from build123d import *

# Parameters (mm, degrees)
SKETCH_1_R      = 7.75
SKETCH_1_R_2    = 1.15
EXTRUDE_1_DEPTH = 11
EXTRUDE_2_DEPTH = 35.9
SKETCH_3_R      = 2
EXTRUDE_3_DEPTH = 10


with BuildPart() as part:
    # 草图1 → 凸台-拉伸1 (new body)
    with BuildSketch(Plane.XY):
        Circle(SKETCH_1_R)
        with Locations((4.353856496, 0)):
            Circle(SKETCH_1_R_2, mode=Mode.SUBTRACT)
        with Locations((-4.646143504, 0)):
            Circle(SKETCH_1_R_2, mode=Mode.SUBTRACT)
    extrude(amount=-EXTRUDE_1_DEPTH)

    # 草图2 → 凸台-拉伸2 (add)
    with BuildSketch(Plane(origin=(0, 0, -11), x_dir=(-1, 0, 0), z_dir=(0, 0, -1))):
        with BuildLine():
            Line((6.5, 4.220485754), (6.5, -4.220485754))
            ThreePointArc((6.5, -4.220485754), (0, -7.75), (-6.5, -4.220485754))
            Line((-6.5, -4.220485754), (-6.5, 4.220485754))
            ThreePointArc((-6.5, 4.220485754), (0, 7.75), (6.5, 4.220485754))
        make_face()
    extrude(amount=EXTRUDE_2_DEPTH)

    # 草图3 → 凸台-拉伸3 (add)
    with BuildSketch(Plane.XY):
        Circle(SKETCH_3_R)
    extrude(amount=EXTRUDE_3_DEPTH)


solid = part.part
Design review of the part built by this model. Coordinates are the model's own, in mm. A direction names the side the tool comes from. Round coordinates to 2 decimals unless told otherwise and drop trailing zeros. Write each loop counter-clockwise with the first axis right and the second up, starting at its lowest first coordinate (ties: lowest second). Pieces come first, ordered by that corner, then holes. Notation, with made-up numbers: (32, 49) - (85, 49) arc R23 ccw to (85, 87) - close; hole circle Ø6 at (3, 77). An arc over 180 degrees is marked (long way). Return JSON: item names as keys, results as strings. Group by question number.
Item 1: We need section C-C on z = -38. Write out the cut boundary in (x, y).
Item 2: Machinability: for faces 1 (the face through (2, -2, 0)), 2 (the face through (0, 0, -46.9)), 3 (the face through (7, 0, -11)), 4 (the face through (-7, 0, -11)), which of the approach directions +Z, -Z, +X, -X, +Y, -Y give a long, thin tool a straight path to every point of the face, cutting with its end or side? Answer none if there is none.
Item 3: Insertion check: P1, Ø4, axis at x = 0, y = 4.5, coming from the +Z side; P2, Ø0.6, axis at x = -7, y = 1.5, coming from the -Z side; P3, Ø1.5, axis at x = -3.5, z = -32.5, coming from the +Y side; P4, Ø6, axis at y = -1, z = 0.5, coming from the +X side. Each pin has a flat end and moves straight along its axis. Give the tip position at first contact, or say it passes through.
Item 4: We need section D-D on y = 2.5. Write out the cut boundary in (x, z), and give its area (3 significant figures).
Item 5: The part is to be moulded in two halves that separate along X. For faces 5 (the face through (4, 0, -11)), 6 (the face through (0, 0, 10)), 7 (the face through (-6.5, 0, -29)), say which applies: pulls with the +X half, pulls with the -X half, needs draft (parallel to the pull), parting line crosses it, or undercut.
Item 6: For probe 1 along Z at (x, y) = (4.5, -4.5); probe 2 along Y at (x, z) = (4, -4); probe 3 along Z at (x, y) = (-4.25, -0.75), list the stretches that pass through material, from the lowest coordinate up. Write a range as [from, to].
Item 7: We need section A-A on y = 0. Write out the cut boundary in (x, z).
Item 8: We need section B-B on x = 0. Write out the cut boundary in (y, z).
Model answer:
{
 "1": {"outline": "(-6.5, -4.22) arc R7.75 ccw to (6.5, -4.22) - (6.5, 4.22) arc R7.75 ccw to (-6.5, 4.22) - close"},
 "2": {"face 1": "+Z", "face 2": "-Z, +X, -X, +Y, -Y", "face 3": "-Z, +X, +Y, -Y", "face 4": "-Z, -X, +Y, -Y"},
 "3": {"P1": "stops at z = 0", "P2": "stops at z = -11", "P3": "stops at y = 7.25", "P4": "stops at x = 7.75"},
 "4": {"outline": "(-7.34, -11) - (-6.5, -11) - (-6.5, -46.9) - (6.5, -46.9) - (6.5, -11) - (7.34, -11) - (7.34, 0) - (-7.34, 0) - close", "area": "628 mm²"},
 "5": {"face 5": "undercut", "face 6": "needs draft", "face 7": "pulls with the -X half"},
 "6": {"probe 1": "z = [-46.9, 0]", "probe 2": "y = [-6.64, -1.09], [1.09, 6.64]", "probe 3": "z = [-46.9, -11]"},
 "7": {"outline": "(-7.75, -11) - (-6.5, -11) - (-6.5, -46.9) - (6.5, -46.9) - (6.5, -11) - (7.75, -11) - (7.75, 0) - (5.5, 0) - (5.5, -11) - (3.2, -11) - (3.2, 0) - (2, 0) - (2, 10) - (-2, 10) - (-2, 0) - (-3.5, 0) - (-3.5, -11) - (-5.8, -11) - (-5.8, 0) - (-7.75, 0) - close"},
 "8": {"outline": "(-7.75, -46.9) - (7.75, -46.9) - (7.75, 0) - (2, 0) - (2, 10) - (-2, 10) - (-2, 0) - (-7.75, 0) - close"}
}
